The listing builds one solid part. Answer for the finished solid, in the listing's coordinates (mm). A direction names the side the tool comes from. Round coordinates to 2 decimals unless told otherwise and drop trailing zeros. Write each loop counter-clockwise with the first axis right and the second up, starting at its lowest first coordinate (ties: lowest second). Pieces come first, ordered by that corner, then holes.
Item 1: Find section C-C on z = 46.5. Give the vertices of the cut face in (x, y).
Item 2: Find section D-D on z = 9. Give the vertices of the cut face in (x, y).
Item 3: Each of these flat-tipped pins is pushed along its axis until it touches: pin 1 (1.5 mm diameter, centred on y = -41.5, z = 16, fed in from +X); pin 2 (4 mm diameter, centred on x = 16, z = 8, fed in from -Y); pin 3 (10 mm diameter, centred on x = -31.5, z = 26.5, fed in from +Y). Where does it stop, or does it pass through?
Item 4: For a pull along Y with two mould halves and no side action, classify faces 1 (the face through (36.556, 57.338, 27.115)), 2 (the face through (-1, -1, 4)), 3 (the face through (-1, 1, 0)) as +Y half, -Y half, draft (parallel to the pull), parting line (faces both ways), or undercut.
Item 5: Find the intervals of material crossed by probe 1 along Y at (x, z) = (0, 35); probe 2 along Z at (x, y) = (45, 22); probe 3 along X at (y, z) = (58, 35), in increasing order.
Item 6: A tool of negligible diameter and unlimited length cuts with its end or side. For faces 4 (the face through (62, 19.52, 36.75)), 5 (the face through (55, -35, 55)), from which of +Z, -Z, +X, -X, +Y, -Y can it reach the whole face along a straight path? Write none if from no direction.
Item 7: Find section A-A on x = 0. Give the vertices of the cut face in (y, z).
```python
from build123d import *

# Parameters (mm, degrees)
SKETCH_1_R        = 68
SKETCH_1_R_2      = 65
EXTRUDE_1_DEPTH   = 55
SKETCH_2_R        = 68
EXTRUDE_1_2_DEPTH = 4
FILLET_1_R        = 15


with BuildPart() as part:
    # 草图1 → Extrude 1 (new body)
    with BuildSketch(Plane.XY):
        Circle(SKETCH_1_R)
        Circle(SKETCH_1_R_2, mode=Mode.SUBTRACT)
    extrude(amount=EXTRUDE_1_DEPTH)

    # 草图2 → Extrude 1 2 (add)
    with BuildSketch(Plane(origin=(0, 0, 0), x_dir=(-1, 0, 0), z_dir=(0, 0, -1))):
        with Locations(Location((0, 0, 0), (0, 0, 180))):
            Circle(SKETCH_2_R)
    extrude(amount=-EXTRUDE_1_2_DEPTH)

    # 圆角1
    fillet_1_edges = [part.edges().sort_by_distance(p)[0] for p in [
        (-65, 0, 4),
    ]]
    fillet(fillet_1_edges, radius=FILLET_1_R)


solid = part.part
```
Check values:
1. outline: circle Ø136 at (0, 0); hole circle Ø130 at (0, 0)
2. outline: circle Ø136 at (0, 0); hole circle Ø122.36 at (0, 0)
3. pin 1: stops at x = 54.44
3. pin 2: stops at y = -66.54
3. pin 3: stops at y = 62.62
4. face 1: parting line
4. face 2: undercut
4. face 3: draft
5. probe 1: y = -68 to -65, 65 to 68
5. probe 2: z = 0 to 4
5. probe 3: x = -35.5 to -29.34, 29.34 to 35.5
6. face 4: +Z
6. face 5: +Z, +X, -X, +Y, -Y
7. outline: (-68, 0) - (68, 0) - (68, 55) - (65, 55) - (65, 19) arc R15 cw to (50, 4) - (-50, 4) arc R15 cw to (-65, 19) - (-65, 55) - (-68, 55) - close
